Drawing for the job (mm, zero at the part's lowest x, y, z). A direction names the side the tool comes from. Give positions to 0.01 mm unless a question says otherwise; leave off trailing zeros. Loops run counter-clockwise (first coordinate to the right, second up) from the corner with the lowest first, then second, coordinate; pieces in that order, holes last. Notation, with made-up numbers: M 52.25,-14.5 L 79.25,-14.5 A32 ccw 79.25,21.5 Z; hole C -2.75,72 d1. An arc over 180 degrees is marked long. Use CSV: the item, a comma, the result in double quotes. Start each with the question number.
(1) Tool access for the marked faces 1 and 2: list every direction of +Z, -Z, +X, -X, +Y, -Y with a clear straight run to the whole face (end or side of a thin tool).
(2) Wall check: line 1 along X through (y, z) = (17, 16.5); line 2 along Z through (x, y) = (88, 18); line 3 along Z through (x, y) = (69, 11) (1 decimal). Give the ranges that are in metal, low to high. Write a range as from..to.
(3) Slice it at B-B on x = 75.5. List the corners of the cut face in (y, z), and give its area (3 significant figures).
(4) Flat gauge pins, fed straight in: P1, Ø10, axis at y = 5.5, z = 26.5, coming from the -X side; P2, Ø12, axis at x = 77.5, y = 4, coming from the -Z side; P3, Ø11.5, axis at y = 27, z = 22, coming from the -X side. Where does each tip first touch, or does it go through?
(5) Slice it at A-A on y = 19.05. List the corners of the cut face in (x, z), and give its area (3 significant figures).
(6) Slice it at C-C on z = 9. List the corners of the cut face in (x, y).
(7) Two-plate mould, pull along Z, no slides. Class the marked faces 3 and 4: pulls with the +Z half, pulls with the -Z half, needs draft (parallel to the pull), parting line crosses it, or undercut.
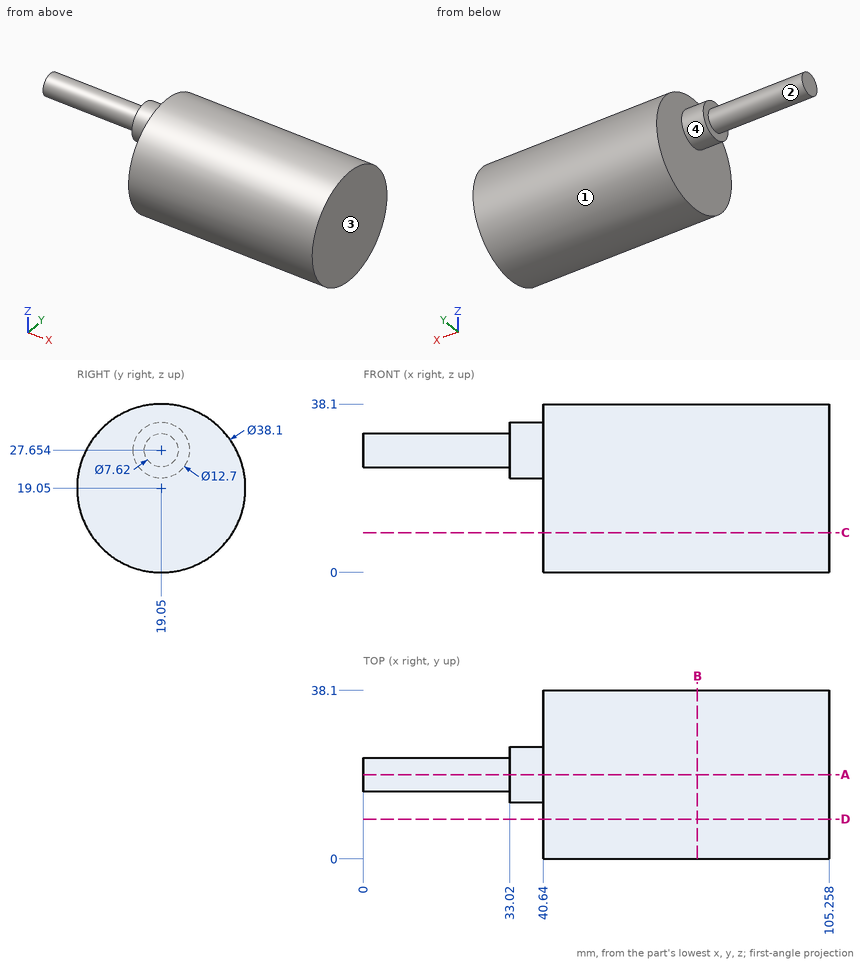
Reply:
1,face 1,"+X, -X"
1,face 2,"-X"
2,line 1,"x = 40.64..105.26"
2,line 2,"z = 0.03..38.07"
2,line 3,"z = 1.8..36.3"
3,outline,"C 19.05,19.05 d38.1"
3,area,"1,140 mm^2"
4,P1,"stops at x = 40.64"
4,P2,"stops at z = 2.29"
4,P3,"stops at x = 33.02"
5,outline,"M 0,23.84 L 33.02,23.84 L 33.02,21.3 L 40.64,21.3 L 40.64,0 L 105.26,0 L 105.26,38.1 L 40.64,38.1 L 40.64,34 L 33.02,34 L 33.02,31.46 L 0,31.46 Z"
5,area,"2,810 mm^2"
6,outline,"M 40.64,2.87 L 105.26,2.87 L 105.26,35.23 L 40.64,35.23 Z"
7,face 3,"needs draft"
7,face 4,"parting line crosses it"
